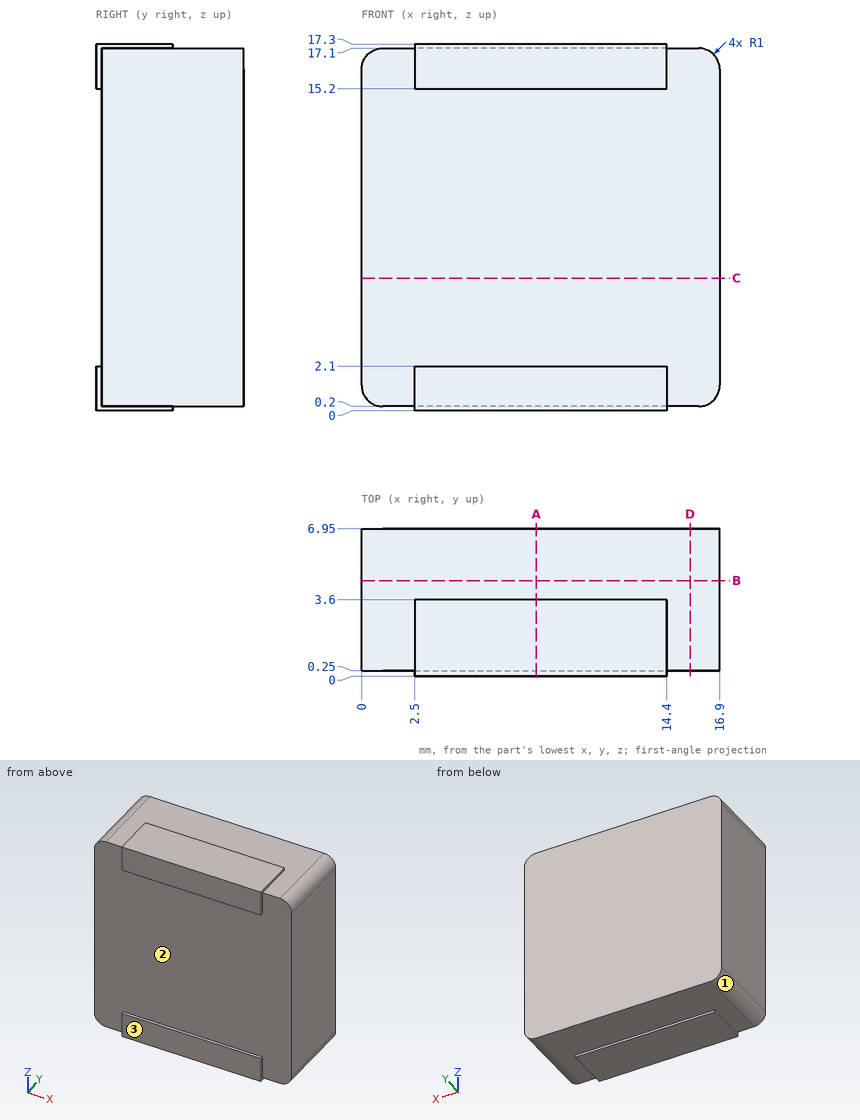
Here's the drawing with two shaded views (mm, measured from the low corner). I have some questions. Round coordinates to 2 decimals unless told otherwise and drop trailing zeros. Order: outer loops, then holes, each group sorted by start corner. A loop starts at its lowest first (then second) coordinate and runs counter-clockwise, first axis right, second up. Notation, with made-up numbers: (39.25, -19.75) -> (90.25, -19.75) arc R23 cw to (90.25, -8.75) -> close; hole circle Ø9 at (-2, 14). An arc over 180 degrees is marked (long way). Use a Markdown table: item, result. Add a question column.
(1) If we mould it in two halves opening along Z, with no side actions, what happens to the marked faces 1, 2 and 3? For each: released by +Z, released by -Z, zero draft, split by the parting line, or undercut.
(2) Suppose I cut it at C-C, the plane z = 6.25. Please give me the cut outline in (x, y).
(3) Suppose I cut it at B-B, the plane y = 4.5. Please give me the cut outline in (x, z).
(4) Suppose I cut it at A-A, the plane x = 8.25. Please give me the cut outline in (y, z).
(5) I need wall thicknesses on line 1 along Y through (x, z) = (15.5, 13.25); line 2 along Z through (x, y) = (12.25, 4). Which ranges of each line are inside material? Lowest first, please.
(6) Suppose I cut it at D-D, the plane x = 15.5. Please give me the cut outline in (y, z), and give its area (3 significant figures).
Verdict:
| question | item | result |
|---|---|---|
| 1 | face 1 | released by -Z |
| 1 | face 2 | undercut |
| 1 | face 3 | zero draft |
| 2 | outline | (0, 0.25) -> (16.9, 0.25) -> (16.9, 6.95) -> (0, 6.95) -> close |
| 3 | outline | (0, 1.2) arc R1 ccw to (1, 0.2) -> (15.9, 0.2) arc R1 ccw to (16.9, 1.2) -> (16.9, 16.1) arc R1 ccw to (15.9, 17.1) -> (1, 17.1) arc R1 ccw to (0, 16.1) -> close |
| 4 | outline | (0, 0) -> (3.6, 0) -> (3.6, 0.2) -> (6.95, 0.2) -> (6.95, 17.1) -> (3.6, 17.1) -> (3.6, 17.3) -> (0, 17.3) -> (0, 15.2) -> (0.25, 15.2) -> (0.25, 2.1) -> (0, 2.1) -> close |
| 5 | line 1 | 0.25 to 6.95 |
| 5 | line 2 | 0.2 to 17.1 |
| 6 | outline | (0.25, 0.2) -> (6.95, 0.2) -> (6.95, 17.1) -> (0.25, 17.1) -> close |
| 6 | area | 113 mm2 |
